Geometry: final body of the model. Coordinates: model frame, mm. A direction names the side the tool comes from. Coordinates: 2 decimals unless noted, no trailing zeros. Write each loop counter-clockwise with the first axis right and the second up, starting at its lowest first coordinate (ties: lowest second). Pieces come first, ordered by that corner, then holes. Notation, with made-up numbers: (78, -29.5) - (126, -29.5) arc R19 cw to (126, -9.5) - close; hole circle Ø8 at (-26.5, 42.25). An arc over 180 degrees is marked (long way). Put each result on its own line as item: value.
```python
from build123d import *

# Parameters (mm, degrees)
SKETCH1_W           = 25
SKETCH1_H           = 40
SKETCH1_R           = 1.75
BOSS_EXTRUDE1_DEPTH = 5
SKETCH2_W           = 3
SKETCH2_H           = 40
BOSS_EXTRUDE2_DEPTH = 0.6
SKETCH3_R           = 3
CUT_EXTRUDE1_DEPTH  = 3


with BuildPart() as part:
    # Sketch1 → Boss-Extrude1 (new body)
    with BuildSketch(Plane.XY):
        with Locations((12.5, 20)):
            Rectangle(SKETCH1_W, SKETCH1_H)
        with Locations((17, 32.5)):
            Circle(SKETCH1_R, mode=Mode.SUBTRACT)
        with Locations((17, 7.5)):
            Circle(SKETCH1_R, mode=Mode.SUBTRACT)
    extrude(amount=BOSS_EXTRUDE1_DEPTH)

    # Sketch2 → Boss-Extrude2 (add)
    with BuildSketch(Plane.XY.offset(5)):
        with Locations((23.5, 20)):
            Rectangle(SKETCH2_W, SKETCH2_H)
    extrude(amount=BOSS_EXTRUDE2_DEPTH)

    # Sketch3 → Cut-Extrude1 (cut)
    with BuildSketch(Plane(origin=(0, 0, 0), x_dir=(-1, 0, 0), z_dir=(0, 0, -1))):
        with Locations((-17, 7.5)):
            Circle(SKETCH3_R)
        with Locations((-17, 32.5)):
            Circle(SKETCH3_R)
    extrude(amount=-CUT_EXTRUDE1_DEPTH, mode=Mode.SUBTRACT)


solid = part.part
```
1. Set-up query: faces 1 (the cylindrical face through (17.9, 34, 4)), 2 (the flat face through (11, 20, 5)), 3 (the flat face through (17, 5.5, 3)). Return all of +Z, -Z, +X, -X, +Y, -Y with unobstructed straight access to the full face (end or side cutting, diameter ignored); none if empty.
Answer below:
face 1: +Z, -Z
face 2: +Z, -X, +Y, -Y
face 3: -Z
2. Mould query, pull axis X, two halves, no side actions, for faces 4 (the cylindrical face through (19.21, 34.53, 1.48)), 5 (the flat face through (17, 30.5, 3)), 6 (the flat face through (12, 0, 3)), 7 (the flat face through (0, 20, 2)). Classes: +X half, -X half, draft (parallel to the pull), parting line (faces both ways), or undercut.
Answer below:
face 4: undercut
face 5: undercut
face 6: draft
face 7: -X half
3. Section query C-C (z = 4.25). Return loops of the section in (x, y), then the cut area to 3 significant figures.
Answer below:
outline: (0, 0) - (25, 0) - (25, 40) - (0, 40) - close; hole circle Ø3.5 at (17, 7.5); hole circle Ø3.5 at (17, 32.5)
area: 981 mm²
4. Section query A-A (x = 17). Return loops of the section in (y, z), then the cut area to 3 significant figures.
Answer below:
outline: (0, 0) - (4.5, 0) - (4.5, 3) - (5.75, 3) - (5.75, 5) - (0, 5) - close; (9.25, 3) - (10.5, 3) - (10.5, 0) - (29.5, 0) - (29.5, 3) - (30.75, 3) - (30.75, 5) - (9.25, 5) - close; (34.25, 3) - (35.5, 3) - (35.5, 0) - (40, 0) - (40, 5) - (34.25, 5) - close
area: 150 mm²
5. Pin query (flat end, axial travel): pin 1 Ø5 at (x, y) = (20, 32.5) entering from +Z; pin 2 Ø1.8 at (x, y) = (18, 31.5) entering from -Z; pin 3 Ø11 at (x, y) = (6, 24) entering from +Z. Return the tip coordinate at first contact, or that it passes through.
Answer below:
pin 1: stops at z = 5.6
pin 2: stops at z = 3
pin 3: stops at z = 5
6. Ray query, probe 1 along Y at (x, z) = (17, 2.4); probe 2 along Y at (x, z) = (17, 4.1); probe 3 along X at (y, z) = (7.5, 3.95). Return the intervals inside material, ascending. Write a range as from..to.
Answer below:
probe 1: y = 0..4.5, 10.5..29.5, 35.5..40
probe 2: y = 0..5.75, 9.25..30.75, 34.25..40
probe 3: x = 0..15.25, 18.75..25
7. Section query B-B (y = 7.5). Return loops of the section in (x, z).
Answer below:
outline: (0, 0) - (14, 0) - (14, 3) - (15.25, 3) - (15.25, 5) - (0, 5) - close; (18.75, 3) - (20, 3) - (20, 0) - (25, 0) - (25, 5.6) - (22, 5.6) - (22, 5) - (18.75, 5) - close
8. Section query D-D (y = 20). Return loops of the section in (x, z), then the cut area to 3 significant figures.
Answer below:
outline: (0, 0) - (25, 0) - (25, 5.6) - (22, 5.6) - (22, 5) - (0, 5) - close
area: 127 mm²
